Source: CAD feature listing. Evaluate the final solid. Frame: model axes, mm. Face numbers are marked on the shaded views. A direction names the side the tool comes from. Give positions to 0.01 mm unless a question says otherwise; leave off trailing zeros. Loops run counter-clockwise (first coordinate to the right, second up) from the corner with the lowest first, then second, coordinate; pieces in that order, holes last. Notation, with made-up numbers: M -5,42.25 L 5,42.25 A6 ccw 5,50.25 Z; hole C 60.25,25.5 d7. An arc over 180 degrees is marked long. Put each result on its own line as item: value.
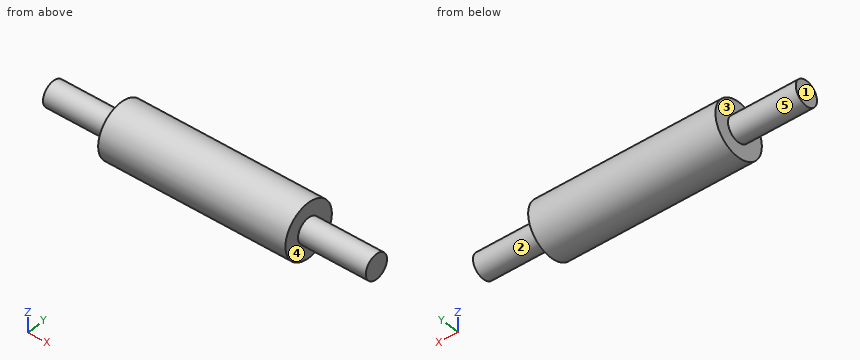
from build123d import *


with BuildPart() as part:
    # Sketch1 → Revolve1 (revolve)
    with BuildSketch(Plane.XY, mode=Mode.PRIVATE) as revolve1_sk:
        Polygon((0, 1.5875), (0, 0.725), (-4, 0.725), (-4, 0), (15.05, 0), (15.05, 0.725), (11.05, 0.725), (11.05, 1.5875), align=None)
    revolve(revolve1_sk.sketch.rotate(Axis((-19.47872402, 0, 0), (1, 0, 0)), 90), axis=Axis((-19.47872402, 0, 0), (1, 0, 0)))  # turned: the seam where the file's is


solid = part.part
1. Section query D-D (y = 1.3). Output: boundary loops of the cut face in (x, z).
Found:
outline: M 0,-0.91 L 11.05,-0.91 L 11.05,0.91 L 0,0.91 Z
2. Draft query along X for the marked faces 3, 4 and 5. Return one class per face: pulls with the +X half, pulls with the -X half, needs draft (parallel to the pull), parting line crosses it, or undercut.
Found:
face 3: pulls with the -X half
face 4: pulls with the +X half
face 5: needs draft
3. Access query for the marked faces 1 and 2. Directions: +Z, -Z, +X, -X, +Y, -Y. A direction counts if a zero-diameter tool reaches every point of the face in a straight line with its end or side. Return the directions, or none.
Found:
face 1: +Z, -Z, -X, +Y, -Y
face 2: +X
4. Section query C-C (x = 9.5). Output: boundary loops of the cut face in (y, z) (1 decimal).
Found:
outline: C 0,0 d3.2
5. Contact query for flat-ended pins moving along their axis: P1, Ø1, axis at y = -1, z = -1, coming from the -X side; P2, Ø1.5, axis at x = 0.5, z = 1, coming from the -Y side; P3, Ø1, axis at y = 1, z = -1, coming from the +X side. Output: stop coordinate, or through.
Found:
P1: x = 0
P2: y = -1.57
P3: x = 11.05
6. Material intervals for line 1 (X direction, y = -0.9, z = 0.7); line 2 (Y direction, x = 7.25, z = -1.1); line 3 (Z direction, x = 5, y = -0.7), sorted ascending. Write a range as from..to.
Found:
line 1: 0..11.05
line 2: -1.14..1.14
line 3: -1.42..1.42
